Verification items for the finished model (mm, model axes). A direction names the side the tool comes from. Round coordinates to 2 decimals unless told otherwise and drop trailing zeros. Write each loop counter-clockwise with the first axis right and the second up, starting at its lowest first coordinate (ties: lowest second). Pieces come first, ordered by that corner, then holes. Notation, with made-up numbers: M -14,41 L 34,41 A25 ccw 34,69 Z; hole C 85.25,84 d1. An arc over 180 degrees is marked long. Use a Markdown table: item, result. Add a question column.
Autodesk Inventor part; units mm, degrees
ref_plane "YZ Plane" through (0, 0, 0) normal (1, 0, 0) x (0, 1, 0)
ref_plane "XZ Plane" through (0, 0, 0) normal (0, 1, 0) x (-1, 0, 0)
ref_plane "XY Plane" through (0, 0, 0) normal (0, 0, 1) x (1, 0, 0)
sketch "Эскиз1" plane through (0, 0, 0) normal (0, 1, 0) x (-1, 0, 0)
  line L0 (0, 0) -> (12.5, 0)
  line L1 (12.5, 0) -> (16.5, 0)
  line L2 (16.5, 0) -> (16.5, -24)
  line L3 (12.5, 0) -> (12.5, -24)
  line L4 (12.5, -24) -> (16.5, -24)
  line L5 (12.5, -24) -> (0, -24)
  line L6 (0, -24) -> (0, -34)
  line L7 (0, -34) -> (17.5, -34)
  line L8 (17.5, -34) -> (17.5, -24)
  line L9 (17.5, -24) -> (16.5, -24)
  line L10 (17.5, -34) -> (21.5, -34)
  line L11 (21.5, -34) -> (21.5, -20)
  line L12 (21.5, -20) -> (16.5, -20)
  dimension "d0" = 12.5
  dimension "d1" = 4
  dimension "d2" = 24
  dimension "d3" = 10
  dimension "d4" = 17.5
  dimension "d5" = 4
  dimension "d6" = 14
revolve "Вращение1" add sketch "Эскиз1" angle 360 about axis through (0, 0, -24) along (0, 0, -1) contours L1 L2 L4 L3 | L12 L11 L10 L8 L9 L2
sketch "Эскиз2" plane through (0, 0, 0) normal (1, 0, 0) x (0, 1, 0)
  line L0 (0, 0) -> (0, -10)
  line L1 (-17.5, -34) -> (17.5, -34)
  line L2 (0, -34) -> (0, -24)
  line L3 (0, -24) -> (0, -29)
  circle A0 centre (0, -10) radius 1.5
  circle A1 centre (0, -29) radius 1.5
  dimension "d8" = 10
  dimension "d9" = 10
  dimension "d10" = 5
  dimension "d11" = 3
  dimension "d12" = 3
extrude "Выдавливание1" cut sketch "Эскиз2" along normal blind 29.75 and the other way blind 30.75
thread "Резьба1"
thread "Резьба2"
properties part number "17701729.303511.017"
1. Cross-section at D-D on y = 8.5. Enter the section's corners in (x, z).
2. Scan lines: line 1 along Z through (x, y) = (-15.6, 0); line 2 along Y through (x, z) = (0, -29.5); line 3 along Z through (x, y) = (10.5, 16). Record each from-to range of solid material in increasing order. Write a range as from..to.
3. Release check for a two-part mould opening along X. For faces 1 (the flat face through (-3.1, -17.4, -34)), 2 (the flat face through (-11, -8, -24)), 3 (the cylindrical face through (-16.166, 6.703, -28.93)), 4 (the cylindrical face through (-15.738, 4.956, -10.14)) record: +X half, -X half, draft (parallel to the pull), parting line (faces both ways), or undercut.
4. Cross-section at B-B on y = 0. Count the separate pieces of the cut face and the enclosed holes in it, plus the area to 3 significant figures.
5. Cross-section at A-A on x = 0. Enter the section's corners in (y, z), plus the area to 3 significant figures.
6. Depth check by flat-ended pin: pin 1 Ø4 at (x, z) = (9.5, -22) entering from +Y; pin 2 Ø8 at (x, z) = (6.5, -8.5) entering from +Y; pin 3 Ø2.5 at (y, z) = (0, -29) entering from +X; pin 4 Ø4 at (y, z) = (0, -10) entering from +X. Enter the tip coordinate at first touch or a pass-through.
7. Cross-section at C-C on z = -22.5. Enter the section's corners in (x, y), plus the area to 3 significant figures.
8. Access from +Z, -Z, +X, -X, +Y, -Y to the whole of each face (thin tool, end or side, straight path). Record for faces 5 (the flat face through (5, -16, -20)), 6 (the cylindrical face through (-19.439, -0.195, -27.513)).
Answer:
| question | item | result |
|---|---|---|
| 1 | outline | M -19.75,-34 L -15.3,-34 L -15.3,-24 L -9.17,-24 L -9.17,0 L -14.14,0 L -14.14,-20 L -19.75,-20 Z; M 9.17,-24 L 15.3,-24 L 15.3,-34 L 19.75,-34 L 19.75,-20 L 14.14,-20 L 14.14,0 L 9.17,0 Z |
| 2 | line 1 | z = -24..-11.5, -8.5..0 |
| 2 | line 2 | y = -21.5..-17.5, 17.5..21.5 |
| 2 | line 3 | z = -34..-20 |
| 3 | face 1 | draft |
| 3 | face 2 | undercut |
| 3 | face 3 | undercut |
| 3 | face 4 | parting line |
| 4 | separate pieces | 6 |
| 4 | enclosed holes | 0 |
| 4 | area | 264 mm^2 |
| 5 | outline | M -21.5,-34 L -17.5,-34 L -17.5,-24 L -12.5,-24 L -12.5,0 L -16.5,0 L -16.5,-20 L -21.5,-20 Z; M 12.5,-24 L 17.5,-24 L 17.5,-34 L 21.5,-34 L 21.5,-20 L 16.5,-20 L 16.5,0 L 12.5,0 Z |
| 5 | area | 312 mm^2 |
| 6 | pin 1 | stops at y = 20.15 |
| 6 | pin 2 | stops at y = 16.31 |
| 6 | pin 3 | passes through |
| 6 | pin 4 | stops at x = 16.5 |
| 7 | outline | C 0,0 d43; hole C 0,0 d25 |
| 7 | area | 961 mm^2 |
| 8 | face 5 | +Z |
| 8 | face 6 | +X, -X |
